Autodesk Inventor part; units mm, degrees
ref_plane "YZ Plane" through (0, 0, 0) normal (1, 0, 0) x (0, 1, 0)
ref_plane "XZ Plane" through (0, 0, 0) normal (0, 1, 0) x (-1, 0, 0)
ref_plane "XY Plane" through (0, 0, 0) normal (0, 0, 1) x (1, 0, 0)
sketch "Sketch1" plane through (0, 0, 0) normal (0, 1, 0) x (-1, 0, 0)
  line L0 (42.5, 33.5) -> (-42.5, 33.5)
  line L1 (-42.5, 33.5) -> (-42.5, -33.5)
  line L2 (-42.5, -33.5) -> (42.5, -33.5)
  line L3 (42.5, -33.5) -> (42.5, 33.5)
  point P0 (0, 0)
  point P1 (42.5, 0)
  point P2 (0, 33.5)
  dimension "d0" = 67
  dimension "d1" = 85
extrude "Extrusion1" add sketch "Sketch1" along normal blind 1
sketch "Sketch2" plane through (0, 1, 0) normal (0, 1, 0) x (1, 0, 0)
  line L0 (-42.5, 33.5) -> (-42.5, -33.5)
  line L1 (42.5, -33.5) -> (42.5, 33.5)
  line L2 (-42.5, -33.5) -> (42.5, -33.5)
  line L3 (42.5, -33.5) -> (42.5, -32.5)
  line L4 (42.5, -32.5) -> (-42.5, -32.5)
  line L5 (-42.5, -32.5) -> (-42.5, -33.5)
  line L6 (-42.5, 32.5) -> (42.5, 32.5)
  line L7 (42.5, 32.5) -> (42.5, 33.5)
  line L8 (42.5, 33.5) -> (-42.5, 33.5)
  line L9 (-42.5, 33.5) -> (-42.5, 32.5)
  point P0 (0, 0)
  dimension "d4" = 1
  dimension "d5" = 1
extrude "Extrusion2" add sketch "Sketch2" along normal blind 10 and the other way blind 11 contours L8 L1 L6 L0 | L4 L1 L2 L0
sketch "Sketch3" plane through (0, 0, 0) normal (0, -1, 0) x (1, 0, 0)
  line L0 (-42.5, -32.5) -> (-42.5, 32.5)
  line L1 (-42.5, -32.5) -> (42.5, -32.5)
  line L2 (-42.5, 32.5) -> (-41.5, 32.5)
  line L3 (-41.5, 32.5) -> (-41.5, -32.5)
  line L4 (-41.5, -32.5) -> (-42.5, -32.5)
  line L5 (-42.5, -32.5) -> (-42.5, 32.5)
  point P0 (0, 0)
  dimension "d10" = 1
extrude "Extrusion3" add sketch "Sketch3" along normal blind 10 and the other way blind 11
sketch "Sketch4" plane through (0, 0, 0) normal (0, -1, 0) x (1, 0, 0)
  line L0 (-2.5, -24.5) -> (-11.5, -24.5)
  line L1 (-11.5, -24.5) -> (-11.5, -27.5)
  line L2 (-11.5, -27.5) -> (-2.5, -27.5)
  line L3 (-2.5, -27.5) -> (-2.5, -24.5)
  line L4 (42.5, -32.5) -> (-41.5, -32.5)
  line L5 (-41.5, -32.5) -> (-41.5, 32.5)
  line L6 (37.5, 6) -> (34.5, 6)
  line L7 (34.5, 6) -> (34.5, -6)
  line L8 (34.5, -6) -> (37.5, -6)
  line L9 (37.5, -6) -> (37.5, 6)
  line L10 (42.5, 32.5) -> (42.5, -32.5)
  line L11 (11.5, 10.5) -> (7.5, 10.5)
  line L12 (7.5, 10.5) -> (7.5, 5.5)
  line L13 (7.5, 5.5) -> (11.5, 5.5)
  line L14 (11.5, 5.5) -> (11.5, 10.5)
  line L15 (-21.5, 10.5) -> (-25.5, 10.5)
  line L16 (-25.5, 10.5) -> (-25.5, 5.5)
  line L17 (-25.5, 5.5) -> (-21.5, 5.5)
  line L18 (-21.5, 5.5) -> (-21.5, 10.5)
  point P0 (0, 0)
  point P1 (37.5, 0)
  dimension "d13" = 9
  dimension "d14" = 3
  dimension "d15" = 5
  dimension "d16" = 30
  dimension "d17" = 12
  dimension "d18" = 3
  dimension "d19" = 5
  dimension "d24" = 5
  dimension "d25" = 4
  dimension "d26" = 5
  dimension "d27" = 4
  dimension "d28" = 10
  dimension "d29" = 10
  dimension "d30" = 30
  dimension "d31" = 30
extrude "Extrusion4" cut sketch "Sketch4" against normal blind 10
properties part number "Thermometer Cover"
Geometry check sheet. Reference: the model listing, model coordinates, mm. A direction names the side the tool comes from. Round coordinates to 2 decimals unless told otherwise and drop trailing zeros. Order: outer loops, then holes, each group sorted by start corner. A loop starts at its lowest first (then second) coordinate and runs counter-clockwise, first axis right, second up. Notation, with made-up numbers: M 55.25,20.25 L 97.25,20.25 A28 ccw 97.25,57.25 Z; hole C 88.25,-19.5 d9. An arc over 180 degrees is marked long. Answer in a Markdown table with one row per item. Add a question column.
Item 1: Draft check along Z on faces 1 (the face through (-41.5, 6, 0)), 2 (the face through (-42.5, 0, 0)), 3 (the face through (1, 0, -33.5)). Enter one of: released by +Z, released by -Z, zero draft, split by the parting line, or undercut.
Item 2: Depth check by flat-ended pin: pin 1 Ø8 at (x, z) = (-17, 6.5) entering from +Y; pin 2 Ø3 at (x, z) = (-3.5, -10.5) entering from -Y; pin 3 Ø3 at (y, z) = (6, -6.5) entering from +X. Enter the tip coordinate at first touch or a pass-through.
Item 3: Sectioned sample at C-C, the plane y = 8.75. Enter the section's corners in (x, z).
Item 4: Material ranges on L1, parallel to Z at x = -4, y = 9.75; L2, parallel to Y at x = 18, z = -8.5; L3, parallel to X at y = 4.75, z = 31, recorded low to high. Write a range as [from, to].
Item 5: Sectioned sample at A-A, the plane z = 8. Enter the section's corners in (x, y), plus the area to 3 significant figures.
Item 6: Sectioned sample at B-B, the plane x = -4. Enter the section's corners in (y, z), plus the area to 3 significant figures.
Item 7: Sectioned sample at D-D, the plane z = -26. Enter the section's corners in (x, y).
Item 8: Set-up check for faces 4 (the face through (-41.5, -5, 0)), 5 (the face through (1, 1, 0)), 6 (the face through (-1, 0, 33.5)): record each of +Z, -Z, +X, -X, +Y, -Y from which the full face is reachable in a straight line by a thin tool's end or side.
Filled in:
| question | item | result |
|---|---|---|
| 1 | face 1 | undercut |
| 1 | face 2 | zero draft |
| 1 | face 3 | released by -Z |
| 2 | pin 1 | stops at y = 1 |
| 2 | pin 2 | stops at y = 0 |
| 2 | pin 3 | stops at x = -41.5 |
| 3 | outline | M -42.5,-33.5 L 42.5,-33.5 L 42.5,-32.5 L -41.5,-32.5 L -41.5,32.5 L 42.5,32.5 L 42.5,33.5 L -42.5,33.5 Z |
| 4 | L1 | z = [-33.5, -32.5], [32.5, 33.5] |
| 4 | L2 | y = [0, 1] |
| 4 | L3 | x = [-42.5, -41.5] |
| 5 | outline | M -42.5,-10 L -41.5,-10 L -41.5,0 L -25.5,0 L -25.5,1 L -41.5,1 L -41.5,11 L -42.5,11 Z; M -21.5,0 L 7.5,0 L 7.5,1 L -21.5,1 Z; M 11.5,0 L 42.5,0 L 42.5,1 L 11.5,1 Z |
| 5 | area | 97.0 mm² |
| 6 | outline | M -10,-33.5 L 11,-33.5 L 11,-32.5 L 1,-32.5 L 1,-27.5 L 0,-27.5 L 0,-32.5 L -10,-32.5 Z; M -10,32.5 L 0,32.5 L 0,-24.5 L 1,-24.5 L 1,32.5 L 11,32.5 L 11,33.5 L -10,33.5 Z |
| 6 | area | 104 mm² |
| 7 | outline | M -42.5,-10 L -41.5,-10 L -41.5,0 L -11.5,0 L -11.5,1 L -41.5,1 L -41.5,11 L -42.5,11 Z; M -2.5,0 L 42.5,0 L 42.5,1 L -2.5,1 Z |
| 8 | face 4 | +X, -Y |
| 8 | face 5 | +X, +Y |
| 8 | face 6 | +Z, +X, -X, +Y, -Y |
